```python
from build123d import *

# Parameters (mm, degrees)
BOSS_EXTRUDE1_DEPTH       = 16
CUT_EXTRUDE3_DEPTH        = 11
SKETCH3_R                 = 4
CUT_EXTRUDE1_DEPTH        = 236.155267855
F_8_0MM_DOWEL_HOLE1_D     = 8
F_8_0MM_DOWEL_HOLE1_DEPTH = 12
F_8_0MM_DOWEL_HOLE1_TIP   = 2.403442476


with BuildPart() as part:
    # Sweep1: sweep along a path in Sketch2
    with BuildLine(Plane(origin=(0, 0, 0), x_dir=(0, 0, -1), z_dir=(1, 0, 0))) as sweep1_path:
        Line((150, 92), (-150, 92))
        ThreePointArc((-150, 92), (-165.556349186, 85.556349186), (-172, 70))
        Line((-172, 70), (-172, -70))
        ThreePointArc((-172, -70), (-165.556349186, -85.556349186), (-150, -92))
        Line((-150, -92), (150, -92))
        ThreePointArc((150, -92), (165.556349186, -85.556349186), (172, -70))
        Line((172, -70), (172, 70))
        ThreePointArc((172, 70), (165.556349186, 85.556349186), (150, 92))
    # Sketch1 → Sweep1 (sweep)
    with BuildSketch(Plane.XY):
        Polygon((-3, 96), (-3, 121), (13, 121), (13, 81), (8, 81), (8, 96), align=None)
    sweep(path=sweep1_path.line)

    # Sketch5 → Boss-Extrude1 (add)
    with BuildSketch(Plane(origin=(13, 0, 0), x_dir=(0, 0, -1), z_dir=(1, 0, 0))):
        with BuildLine():
            Line((201, 70), (201, -70))
            ThreePointArc((201, -70), (186.062445841, -106.062445841), (150, -121))
            Line((150, -121), (-150, -121))
            ThreePointArc((-150, -121), (-186.062445841, -106.062445841), (-201, -70))
            Line((-201, -70), (-201, 70))
            ThreePointArc((-201, 70), (-186.062445841, 106.062445841), (-150, 121))
            Line((-150, 121), (150, 121))
            ThreePointArc((150, 121), (186.062445841, 106.062445841), (201, 70))
        make_face()
        with BuildLine():
            Line((-161, -70), (-161, 70))
            ThreePointArc((-161, 70), (-157.778174593, 77.778174593), (-150, 81))
            Line((-150, 81), (150, 81))
            ThreePointArc((150, 81), (157.778174593, 77.778174593), (161, 70))
            Line((161, 70), (161, -70))
            ThreePointArc((161, -70), (157.778174593, -77.778174593), (150, -81))
            Line((150, -81), (-150, -81))
            ThreePointArc((-150, -81), (-157.778174593, -77.778174593), (-161, -70))
        make_face(mode=Mode.SUBTRACT)
    extrude(amount=-BOSS_EXTRUDE1_DEPTH)

    # Sketch6 → Cut-Extrude3 (cut)
    with BuildSketch(Plane.ZY.offset(3)):
        with BuildLine():
            Line((176, -70), (176, 70))
            ThreePointArc((176, 70), (168.384776311, 88.384776311), (150, 96))
            Line((150, 96), (-150, 96))
            ThreePointArc((-150, 96), (-168.384776311, 88.384776311), (-176, 70))
            Line((-176, 70), (-176, -70))
            ThreePointArc((-176, -70), (-168.384776311, -88.384776311), (-150, -96))
            Line((-150, -96), (150, -96))
            ThreePointArc((150, -96), (168.384776311, -88.384776311), (176, -70))
        make_face()
    extrude(amount=-CUT_EXTRUDE3_DEPTH, mode=Mode.SUBTRACT)

    # Sketch3 → Cut-Extrude1 (cut, through all)
    with BuildSketch(Plane(origin=(13, 0, 0), x_dir=(0, 0, -1), z_dir=(1, 0, 0))):
        with Locations(Location((111, 86.5, 0), (0, 0, 90))):
            Circle(SKETCH3_R)
        with Locations(Location((136, 86.5, 0), (0, 0, 90))):
            Circle(SKETCH3_R)
    extrude(amount=-CUT_EXTRUDE1_DEPTH, mode=Mode.SUBTRACT)

    # Ø8.0mm Dowel Hole1
    with Locations(Plane(origin=(-3, 0, -188.5), x_dir=(0, -1, 0), z_dir=(-1, 0, 0))):
        with Locations((0, 0), (0, 377)):
            Hole(F_8_0MM_DOWEL_HOLE1_D / 2, depth=F_8_0MM_DOWEL_HOLE1_DEPTH)
            with Locations((0, 0, -(F_8_0MM_DOWEL_HOLE1_DEPTH + F_8_0MM_DOWEL_HOLE1_TIP / 2))):  # 118° drill point
                Cone(0, F_8_0MM_DOWEL_HOLE1_D / 2, F_8_0MM_DOWEL_HOLE1_TIP, mode=Mode.SUBTRACT)


solid = part.part
```
Here's how the part is built. I have some questions about the finished solid (model axes, mm). A direction names the side the tool comes from. Round coordinates to 2 decimals unless told otherwise and drop trailing zeros. Loops run counter-clockwise (first coordinate to the right, second up) from the corner with the lowest first, then second, coordinate; pieces in that order, holes last. Notation, with made-up numbers: (-6, 70.25) -> (26, 70.25) arc R23 cw to (26, 80.25) -> close; hole circle Ø2 at (-5, 48). An arc over 180 degrees is marked (long way). Answer as CSV lines item,"result".
1. If we section it at B-B on y = 54.5: Please give me the cut outline in (x, z), plus the area to 3 significant figures.
Final values:
outline,"(-3, -201) -> (13, -201) -> (13, -161) -> (8, -161) -> (8, -176) -> (-3, -176) -> close; (-3, 176) -> (8, 176) -> (8, 161) -> (13, 161) -> (13, 201) -> (-3, 201) -> close"
area,"950 mm^2"
2. If we section it at A-A on z = -111: Please give me the cut outline in (x, y), plus the area to 3 significant figures.
Final values:
outline,"(-3, -121) -> (13, -121) -> (13, -81) -> (8, -81) -> (8, -96) -> (-3, -96) -> close; (-3, 96) -> (8, 96) -> (8, 90.5) -> (13, 90.5) -> (13, 121) -> (-3, 121) -> close; (8, 81) -> (13, 81) -> (13, 82.5) -> (8, 82.5) -> close"
area,"910 mm^2"
3. If we section it at D-D on y = 86.5: Please give me the cut outline in (x, z), plus the area to 3 significant figures.
Final values:
outline,"(-3, -198.26) -> (13, -198.26) -> (13, -140) -> (8, -140) -> (8, -170.09) -> (-3, -170.09) -> close; (-3, 170.09) -> (8, 170.09) -> (8, -107) -> (13, -107) -> (13, 198.26) -> (-3, 198.26) -> close; (8, -132) -> (13, -132) -> (13, -115) -> (8, -115) -> close"
area,"2,520 mm^2"
4. Which directions (+Z, -Z, +X, -X, +Y, -Y) give clear straight access to the entire face, cutting with the end or side of a thin tool? Please do faces 4 (the face through (10.535, 77.863, 157.692)), 5 (the face through (5, 121, 2)), 6 (the face through (8, 86, -14)).
Final values:
face 4,"+X, -X"
face 5,"+Z, -Z, +X, -X, +Y"
face 6,"-X"
5. If I drill on L1, parallel to Z at x = 4.25, y = 0; L2, parallel to Z at x = 2.25, y = -30; L3, parallel to Y at x = 9.5, z = 29.5, over which ranges is the centre line in solid material (lowest first)?
Final values:
L1,"z = -201 to -192.5, -184.5 to -176, 176 to 184.5, 192.5 to 201"
L2,"z = -201 to -176, 176 to 201"
L3,"y = -121 to -81, 81 to 121"
6. Thinking about a two-plate mould opening in Y: for faces 1 (the face through (5, -121, -2)), 2 (the face through (4.89, 106.46, 185.66)), 3 (the face through (2.42, 88.18, 168.59)), which applies, released by +Y, released by -Y, zero draft, split by the parting line, or undercut?
Final values:
face 1,"released by -Y"
face 2,"released by +Y"
face 3,"undercut"
7. For pin 1 (7 mm diameter, centred on y = 86.5, z = -136, fed in from -X); pin 2 (12 mm diameter, centred on y = 86, z = -50.5, fed in from -X); pin 3 (5 mm diameter, centred on y = 0, z = -188.5, fed in from -X), each with a flat end and sliding along its axis, tell me the tip position at first contact or that it passes through.
Final values:
pin 1,"passes through"
pin 2,"stops at x = 8"
pin 3,"stops at x = 9.9"
8. If we section it at C-C on x = 0: Please give me the cut outline in (y, z).
Final values:
outline,"(-121, -150) arc R51 ccw to (-70, -201) -> (70, -201) arc R51 ccw to (121, -150) -> (121, 150) arc R51 ccw to (70, 201) -> (-70, 201) arc R51 ccw to (-121, 150) -> close; hole (-96, -150) arc R26 ccw to (-70, -176) -> (70, -176) arc R26 ccw to (96, -150) -> (96, 150) arc R26 ccw to (70, 176) -> (-70, 176) arc R26 ccw to (-96, 150) -> close; hole circle Ø8 at (0, -188.5); hole circle Ø8 at (0, 188.5)"
